from build123d import *

# Parameters (mm, degrees)
F0_W     = 69.5
F0_H     = 40
F0_R     = 1.5
F0_R_2   = 0.75
F0_W_2   = 42
F0_H_2   = 21.5
F1_DEPTH = 3
F3_R     = 3


with BuildPart() as f1:
    # F0 (on Top) → F1 (new body)
    with BuildSketch(Plane.XY):
        Rectangle(F0_W, F0_H)
        with Locations((-29.75, -15)):
            Circle(F0_R, mode=Mode.SUBTRACT)
        with Locations((-24.75, -5)):
            Circle(F0_R_2, mode=Mode.SUBTRACT)
        with Locations((29.75, -15)):
            Circle(F0_R, mode=Mode.SUBTRACT)
        with Locations((24.75, -5)):
            Circle(F0_R_2, mode=Mode.SUBTRACT)
        with Locations((-24.75, 5)):
            Circle(F0_R_2, mode=Mode.SUBTRACT)
        with Locations((-29.75, 15)):
            Circle(F0_R, mode=Mode.SUBTRACT)
        Rectangle(F0_W_2, F0_H_2, mode=Mode.SUBTRACT)
        with Locations((24.75, 5)):
            Circle(F0_R_2, mode=Mode.SUBTRACT)
        with Locations((29.75, 15)):
            Circle(F0_R, mode=Mode.SUBTRACT)
    extrude(amount=F1_DEPTH)

    # F2: F1 across face


with BuildPart() as f1_1:
    add(f1.part)
    add(f1.part.mirror(Plane(origin=(0, -20, 1.5), x_dir=(1, 0, 0), z_dir=(0, -1, 0))))

    # F3
    f3_edges = [f1_1.edges().sort_by_distance(p)[0] for p in [
        (-34.75, -60, 1.5),
        (34.75, -60, 1.5),
        (34.75, 20, 1.5),
        (-34.75, 20, 1.5),
    ]]
    fillet(f3_edges, radius=F3_R)


solid = f1_1.part
Check sheet for the modelled part. Datum: model origin and axes. Units: mm. A direction names the side the tool comes from. Give positions to 0.01 mm unless a question says otherwise; leave off trailing zeros. Write each loop counter-clockwise with the first axis right and the second up, starting at its lowest first coordinate (ties: lowest second). Pieces come first, ordered by that corner, then holes. Notation, with made-up numbers: (61, 89) -> (82, 89) arc R20 ccw to (82, 114) -> close; hole circle Ø10 at (-9, 51.5). An arc over 180 degrees is marked (long way). Use one line per item in the form item = value. Start each with the question number.
1. Section check A-A (y = -15). Record the cut outline in (x, z), and give its area (4 significant figures).
2. Mould release check, pull along X, two halves, no side actions. Record for faces 1 (the flat face through (-21, -40, 1)), 2 (the cylindrical face through (33.89, 19.1, 1.52)), 3 (the cylindrical face through (-33.89, -59.1, 1.52)): pulls with the +X half, pulls with the -X half, needs draft (parallel to the pull), parting line crosses it, or undercut.
3. Go/stop test with a flat-tipped pin: P1, Ø1.4, axis at x = -24.75, y = -45, coming from the +Z side. Record where the tip stops, or that it passes through.
4. Section check B-B (z = 1.75). Count the separate pieces of the cut face and the enclosed holes in it, and give its area (3 significant figures).
5. Section check D-D (y = -43). Record the cut outline in (x, z).
6. Section check C-C (x = 8). Record the cut outline in (y, z).
7. Thickness scan on line 1 along Y through (x, z) = (29.75, 0.8); line 2 along Y through (x, z) = (16.5, 2.05); line 3 along Y through (x, z) = (-24.75, 1.5). Record the ranges inside material, lowest first. Write a range as from..to.
8. Access from +Z, -Z, +X, -X, +Y, -Y to the whole of each face (thin tool, end or side, straight path). Record for faces 4 (the flat face through (0, 20, 1)), 5 (the flat face through (0, 10.75, 1)).
Conclusion:
q1.outline = (-34.75, 0) -> (-31.25, 0) -> (-31.25, 3) -> (-34.75, 3) -> close; (-28.25, 0) -> (28.25, 0) -> (28.25, 3) -> (-28.25, 3) -> close; (31.25, 0) -> (34.75, 0) -> (34.75, 3) -> (31.25, 3) -> close
q1.area = 190.5 mm²
q2.face_1 = undercut
q2.face_2 = pulls with the +X half
q2.face_3 = pulls with the -X half
q3.P1 = through
q4.separate_pieces = 1
q4.enclosed_holes = 18
q4.area = 3,680 mm²
q5.outline = (-34.75, 0) -> (-21, 0) -> (-21, 3) -> (-34.75, 3) -> close; (21, 0) -> (34.75, 0) -> (34.75, 3) -> (21, 3) -> close
q6.outline = (-60, 0) -> (-50.75, 0) -> (-50.75, 3) -> (-60, 3) -> close; (-29.25, 0) -> (-10.75, 0) -> (-10.75, 3) -> (-29.25, 3) -> close; (10.75, 0) -> (20, 0) -> (20, 3) -> (10.75, 3) -> close
q7.line_1 = -60..-56.5, -53.5..-26.5, -23.5..-16.5, -13.5..13.5, 16.5..20
q7.line_2 = -60..-50.75, -29.25..-10.75, 10.75..20
q7.line_3 = -60..-45.75, -44.25..-35.75, -34.25..-5.75, -4.25..4.25, 5.75..20
q8.face_4 = +Z, -Z, +X, -X, +Y
q8.face_5 = +Z, -Z
